```python
from build123d import *

# Parameters (mm, degrees)
BOSS_EXTRUDE1_DEPTH = 20
SKETCH3_R           = 3
CUT_EXTRUDE1_DEPTH  = 5


with BuildPart() as part:
    # Sketch2 → Boss-Extrude1 (new body)
    with BuildSketch(Plane.XY):
        with BuildLine():
            Line((0, 11.5), (77, 11.5))
            ThreePointArc((77, 11.5), (88.5, 0), (77, -11.5))
            Line((77, -11.5), (0, -11.5))
            ThreePointArc((0, -11.5), (-11.5, 0), (0, 11.5))
        make_face()
    extrude(amount=BOSS_EXTRUDE1_DEPTH)

    # Sketch3 → Cut-Extrude1 (cut)
    with BuildSketch(Plane.XZ.offset(11.5)):
        with Locations((38.5, 10)):
            Circle(SKETCH3_R)
    extrude(amount=-CUT_EXTRUDE1_DEPTH, mode=Mode.SUBTRACT)


solid = part.part
```
The listing builds one solid part. Answer for the finished solid, in the listing's coordinates (mm). A direction names the side the tool comes from. Coordinates: 2 decimals unless noted, no trailing zeros. Loops run counter-clockwise (first coordinate to the right, second up) from the corner with the lowest first, then second, coordinate; pieces in that order, holes last. Notation, with made-up numbers: M 34.25,-27 L 74.25,-27 A15 cw 74.25,-16 Z; hole C 42.5,62 d8. An arc over 180 degrees is marked long. Answer as CSV lines item,"result". Start each with the question number.
(1) Find the intervals of material crossed by L1, parallel to Z at x = 38.5, y = -9.9; L2, parallel to Y at x = 41, z = 10.75; L3, parallel to X at y = 0, z = 16.5, in increasing order. Write a range as [from, to].
(2) The part is cut by section C-C (y = -9). Give the vertices of the cut face in (x, z), and give its area (3 significant figures).
(3) The mould has two halves that part along X. Classify faces 1 (the cylindrical face through (88.497, 0.253, 9.86)), 2 (the cylindrical face through (35.5, -9, 10.1)), 3 (the cylindrical face through (-11.497, -0.253, 9.86)): pulls with the +X half, pulls with the -X half, needs draft (parallel to the pull), parting line crosses it, or undercut.
(4) The part is cut by section B-B (z = 10). Give the vertices of the cut face in (x, y).
(5) Given pin 1 (4 mm diameter, centred on y = 7, z = 3.5, fed in from -X); pin 2 (1.8 mm diameter, centred on x = 37.5, z = 8.5, fed in from -Y); pin 3 (1 mm diameter, centred on y = 2, z = 17.5, fed in from -X), each flat-ended and moving along its own axis, determine where each tip first touches the part or whether it passes through.
(6) For faces 4 (the flat face through (38, -6.5, 10)), 5 (the flat face through (39, -11.5, 5)), determine the directions among +Z, -Z, +X, -X, +Y, -Y from which every point of the face is accessible in a straight line to the end or side of a thin tool.
(7) The part is cut by section A-A (x = 38.5). Give the vertices of the cut face in (y, z), and give its area (3 significant figures).
(8) The part is cut by section D-D (y = 7.25). Give the vertices of the cut face in (x, z).
Determined:
1,L1,"[0, 7], [13, 20]"
1,L2,"[-6.5, 11.5]"
1,L3,"[-11.5, 88.5]"
2,outline,"M -7.16,0 L 84.16,0 L 84.16,20 L -7.16,20 Z; hole C 38.5,10 d6"
2,area,"1,800 mm2"
3,face 1,"pulls with the +X half"
3,face 2,"undercut"
3,face 3,"pulls with the -X half"
4,outline,"M 0,-11.5 L 35.5,-11.5 L 35.5,-6.5 L 41.5,-6.5 L 41.5,-11.5 L 77,-11.5 A11.5 ccw 77,11.5 L 0,11.5 A11.5 ccw Z"
5,pin 1,"x = -10.36"
5,pin 2,"y = -6.5"
5,pin 3,"x = -11.4"
6,face 4,"-Y"
6,face 5,"+Z, -Z, +X, -X, -Y"
7,outline,"M -11.5,0 L 11.5,0 L 11.5,20 L -11.5,20 L -11.5,13 L -6.5,13 L -6.5,7 L -11.5,7 Z"
7,area,"430 mm2"
8,outline,"M -8.93,0 L 85.93,0 L 85.93,20 L -8.93,20 Z"
